For this review, take the finished solid that the model builds, in its own axes (mm). Round coordinates to 2 decimals unless told otherwise and drop trailing zeros. Write each loop counter-clockwise with the first axis right and the second up, starting at its lowest first coordinate (ties: lowest second). Pieces come first, ordered by that corner, then holes. Notation, with made-up numbers: (48.25, 39.5) -> (72.25, 39.5) arc R27 cw to (72.25, 70.5) -> close; hole circle Ø1 at (35, -13). An arc over 180 degrees is marked (long way). Answer in a Markdown table with one row per item.
from build123d import *

# Parameters (mm, degrees)
SKETCH007_W     = 116.5
SKETCH007_H     = 84
PAD002_DEPTH    = 2
SKETCH008_W     = 112.5
SKETCH008_H     = 80
PAD003_DEPTH    = 2
SKETCH009_W     = 108.5
SKETCH009_H     = 76
POCKET004_DEPTH = 2
CHAMFER004_SIZE = 1
FILLET002_R     = 0.5
FILLET003_R     = 1
FILLET004_R     = 1
FILLET005_R     = 1
FILLET006_R     = 1
FILLET007_R     = 0.2


with BuildPart() as part:
    # Sketch007 → Pad002 (new body)
    with BuildSketch(Plane(origin=(0, 0, 0), x_dir=(1, 0, 0), z_dir=(0, 0, -1))):
        with Locations((58.25, 42)):
            Rectangle(SKETCH007_W, SKETCH007_H)
    extrude(amount=PAD002_DEPTH)

    # Sketch008 (on Face5 of Pad002) → Pad003 (new body)
    with BuildSketch(Plane.XY):
        with Locations((58.25, -42)):
            Rectangle(SKETCH008_W, SKETCH008_H)
    extrude(amount=PAD003_DEPTH)

    # Sketch009 (on Face11 of Pad003) → Pocket004 (cut)
    with BuildSketch(Plane.XY.offset(2)):
        with Locations((58.25, -42)):
            Rectangle(SKETCH009_W, SKETCH009_H)
    extrude(amount=-POCKET004_DEPTH, mode=Mode.SUBTRACT)

    # Chamfer004
    chamfer004_edges = [part.edges().sort_by_distance(p)[0] for p in [
        (112.5, -42, 2),
        (58.25, -4, 2),
        (4, -42, 2),
        (58.25, -80, 2),
    ]]
    chamfer(chamfer004_edges, length=CHAMFER004_SIZE)

    # Fillet002
    fillet002_edges = [part.edges().sort_by_distance(p)[0] for p in [
        (58.25, -2, 2),
        (2, -42, 2),
        (114.5, -42, 2),
        (58.25, -82, 2),
    ]]
    fillet(fillet002_edges, radius=FILLET002_R)

    # Fillet003
    fillet003_edges = [part.edges().sort_by_distance(p)[0] for p in [
        (0, 0, -1),
    ]]
    fillet(fillet003_edges, radius=FILLET003_R)

    # Fillet004
    fillet004_edges = [part.edges().sort_by_distance(p)[0] for p in [
        (116.5, 0, -1),
    ]]
    fillet(fillet004_edges, radius=FILLET004_R)

    # Fillet005
    fillet005_edges = [part.edges().sort_by_distance(p)[0] for p in [
        (0, -84, -1),
    ]]
    fillet(fillet005_edges, radius=FILLET005_R)

    # Fillet006
    fillet006_edges = [part.edges().sort_by_distance(p)[0] for p in [
        (116.5, -84, -1),
    ]]
    fillet(fillet006_edges, radius=FILLET006_R)

    # Fillet007
    fillet007_edges = [part.edges().sort_by_distance(p)[0] for p in [
        (114.5, -2, 0.75),
    ]]
    fillet(fillet007_edges, radius=FILLET007_R)


solid = part.part
1) Clearance check with flat-ended pins moving along their axes: pin 1 Ø8 at (x, y) = (74.5, -25.5) entering from +Z; pin 2 Ø0.8 at (y, z) = (-61, 0.5) entering from -X; pin 3 Ø0.5 at (x, z) = (41.5, 0.5) entering from -Y. State where each tip first meets the part, or that it passes through.
Solved:
| item | result |
|---|---|
| pin 1 | z = 0 |
| pin 2 | x = 2 |
| pin 3 | y = -82 |
2) Consider section A-A on y = -73. State the section outline as (x, z) points.
Solved:
| item | result |
|---|---|
| outline | (0, -2) -> (116.5, -2) -> (116.5, 0) -> (114.5, 0) -> (114.5, 1.5) arc R0.5 ccw to (114, 2) -> (113.5, 2) -> (112.5, 1) -> (112.5, 0) -> (4, 0) -> (4, 1) -> (3, 2) -> (2.5, 2) arc R0.5 ccw to (2, 1.5) -> (2, 0) -> (0, 0) -> close |
3) Consider section B-B on x = 70. State the section outline as (y, z) points, then the cut area to 3 significant figures.
Solved:
| item | result |
|---|---|
| outline | (-84, -2) -> (0, -2) -> (0, 0) -> (-2, 0) -> (-2, 1.5) arc R0.5 ccw to (-2.5, 2) -> (-3, 2) -> (-4, 1) -> (-4, 0) -> (-80, 0) -> (-80, 1) -> (-81, 2) -> (-81.5, 2) arc R0.5 ccw to (-82, 1.5) -> (-82, 0) -> (-84, 0) -> close |
| area | 175 mm² |
4) Mouldability with a two-part tool opening along Y and no side actions: class faces 1 (the flat face through (57, -43, -2)), 2 (the flat face through (57, -41, 0)) as pulls with the +Y half, pulls with the -Y half, needs draft (parallel to the pull), parting line crosses it, or undercut.
Solved:
| item | result |
|---|---|
| face 1 | needs draft |
| face 2 | undercut |
5) For line 1 (X direction, y = -74.5, z = 0.9); line 2 (Y direction, x = 55, z = 0.2); line 3 (Z direction, x = 92.5, y = -50), list the stretches that pass through material, from the lowest coordinate up. Write a range as [from, to].
Solved:
| item | result |
|---|---|
| line 1 | [2, 4], [112.5, 114.5] |
| line 2 | [-82, -80], [-4, -2] |
| line 3 | [-2, 0] |
